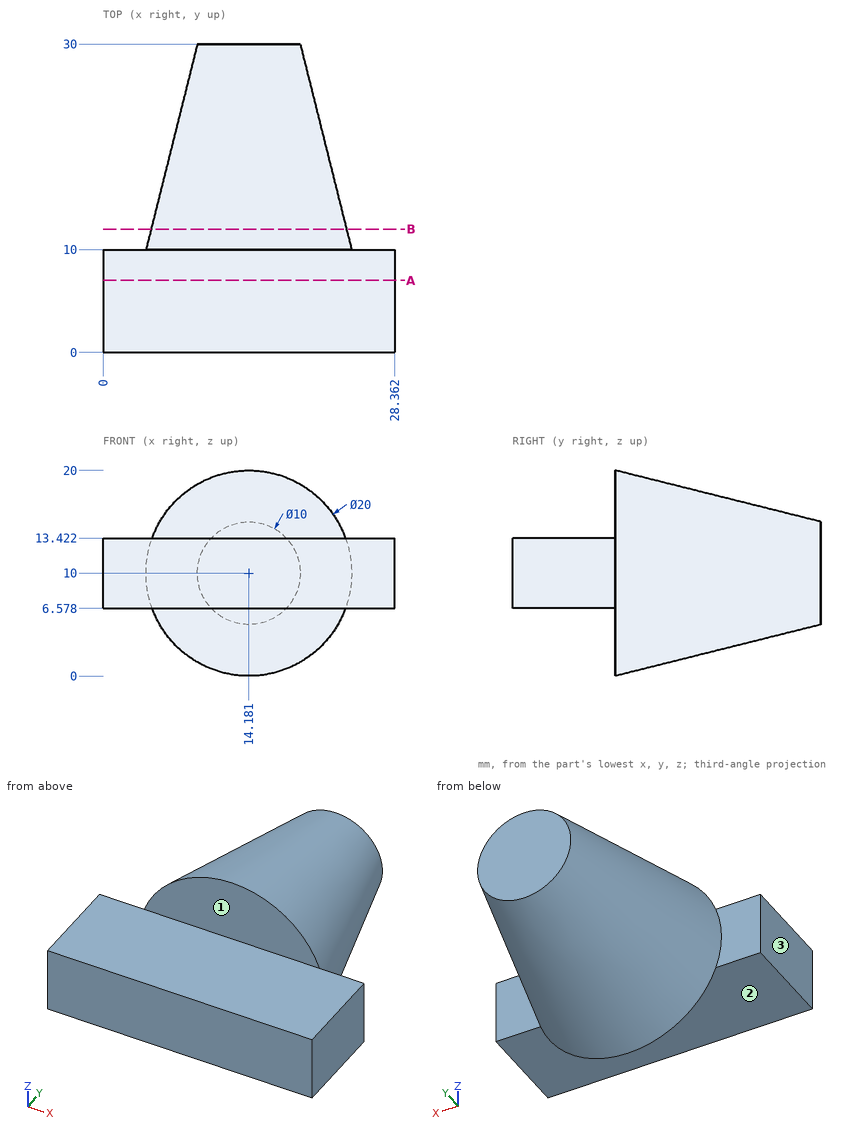
Geometry check sheet. Reference: drawing and pictorial views, mm from the part's lowest x, y, z. A direction names the side the tool comes from. Round coordinates to 2 decimals unless told otherwise and drop trailing zeros. Order: outer loops, then holes, each group sorted by start corner. A loop starts at its lowest first (then second) coordinate and runs counter-clockwise, first axis right, second up. Notation, with made-up numbers: M -18,35 L 27,35 A27 cw 27,58 Z; hole C 54,-35.5 d2. An arc over 180 degrees is marked long. Write item = value, one per line.
Q1. Set-up check for the marked faces 1, 2 and 3: record each of +Z, -Z, +X, -X, +Y, -Y from which the full face is reachable in a straight line by a thin tool's end or side.
Answer block:
face_1 = +Z, +X, -X, -Y
face_2 = -Z, +X, -X, -Y
face_3 = +Z, -Z, -X, +Y, -Y
Q2. Scan lines: line 1 (Z direction, x = 24, y = 5.5); line 2 (Y direction, x = 2.5, z = 10.5); line 3 (Z direction, x = 22, y = 13) (1 decimal). Record each from-to range of solid material in increasing order.
Answer block:
line_1 = 6.58 to 13.42
line_2 = 0 to 10
line_3 = 5.1 to 14.9
Q3. Depth check by flat-ended pin: pin 1 Ø2 at (x, z) = (13.5, 4.5) entering from +Y; pin 2 Ø5 at (x, y) = (16.5, 4) entering from -Z; pin 3 Ø10 at (y, z) = (14, 17.5) entering from +X; pin 4 Ø1 at (y, z) = (25, 9.5) entering from -X. Enter the tip coordinate at first touch or a pass-through.
Answer block:
pin_1 = 30
pin_2 = 6.58
pin_3 = 23.28
pin_4 = 7.82
Q4. Section check A-A (y = 7). Enter the section's corners in (x, z).
Answer block:
outline = M 0,6.58 L 28.36,6.58 L 28.36,13.42 L 0,13.42 Z
Q5. Section check B-B (y = 12). Enter the section's corners in (x, z).
Answer block:
outline = C 14.18,10 d19
